from build123d import *

# Parameters (mm, degrees)
ESQUISSE1_W             = 51.5
ESQUISSE1_H             = 36.5
BOSS_EXTRU_1_DEPTH      = 5
ESQUISSE2_R             = 1.5
ENL_V_MAT_EXTRU_1_DEPTH = 5
ESQUISSE3_W             = 51.5
ESQUISSE3_H             = 2
BOSS_EXTRU_3_DEPTH      = 34.5
ESQUISSE5_R             = 1.5
ESQUISSE5_R_2           = 11
ENL_V_MAT_EXTRU_3_DEPTH = 34.5


with BuildPart() as part:
    # Esquisse1 → Boss.-Extru.1 (new body)
    with BuildSketch(Plane.XY):
        with Locations((11.117800259, -7.384341637)):
            Rectangle(ESQUISSE1_W, ESQUISSE1_H)
    extrude(amount=BOSS_EXTRU_1_DEPTH)

    # Esquisse2 → Enlèv. mat.-Extru.1 (cut)
    with BuildSketch(Plane.XY.offset(5)):
        with Locations((-10.382199741, 4.615658363)):
            Circle(ESQUISSE2_R)
        with Locations((-10.382199741, -21.384341637)):
            Circle(ESQUISSE2_R)
        with Locations((32.617800259, -21.384341637)):
            Circle(ESQUISSE2_R)
        with Locations((32.617800259, 4.615658363)):
            Circle(ESQUISSE2_R)
    extrude(amount=-ENL_V_MAT_EXTRU_1_DEPTH, mode=Mode.SUBTRACT)

    # Esquisse3 → Boss.-Extru.3 (add)
    with BuildSketch(Plane.XY.offset(5)):
        with Locations((11.117800259, 9.865658363)):
            Rectangle(ESQUISSE3_W, ESQUISSE3_H)
    extrude(amount=BOSS_EXTRU_3_DEPTH)

    # Esquisse5 → Enlèv. mat.-Extru.3 (cut)
    with BuildSketch(Plane.XZ.offset(-8.865658363)):
        with Locations((-1.882199741, 35.25)):
            Circle(ESQUISSE5_R)
        with Locations((24.117800259, 35.25)):
            Circle(ESQUISSE5_R)
        with Locations((-1.882199741, 9.25)):
            Circle(ESQUISSE5_R)
        with Locations((24.117800259, 9.25)):
            Circle(ESQUISSE5_R)
        with Locations((11.117800259, 22.25)):
            Circle(ESQUISSE5_R_2)
    extrude(amount=-ENL_V_MAT_EXTRU_3_DEPTH, mode=Mode.SUBTRACT)


solid = part.part
Model file for the job. Use its own axes, mm. A direction names the side the tool comes from. Give positions to 0.01 mm unless a question says otherwise; leave off trailing zeros. Loops run counter-clockwise (first coordinate to the right, second up) from the corner with the lowest first, then second, coordinate; pieces in that order, holes last. Notation, with made-up numbers: (4.25, 67) - (14.25, 67) arc R23 cw to (14.25, 102) - close; hole circle Ø3 at (5, 62.5). An arc over 180 degrees is marked (long way). Use one line per item in the form item = value.
(1) Pull direction X, two halves, no side cores. Call faces 3 (the face through (31.12, -21.32, 2.54)), 4 (the face through (-3.073, 9.852, 8.337)), 5 (the face through (11, -8, 5)), 6 (the face through (36.868, -5, 4)): pulls with the +X half, pulls with the -X half, needs draft (parallel to the pull), parting line crosses it, or undercut.
Determined:
face_3 = undercut
face_4 = undercut
face_5 = needs draft
face_6 = pulls with the +X half
(2) Drill centre lines: L1, parallel to X at y = 4.5, z = 4; L2, parallel to X at y = 4, z = 2; L3, parallel to Z at x = 24, y = -23. Where is each one in solid material? Low to high.
Determined:
L1 = -14.63 to -11.88, -8.89 to 31.12, 34.11 to 36.87
L2 = -14.63 to -11.75, -9.01 to 31.25, 33.99 to 36.87
L3 = 0 to 5
(3) 3-axis set-ups, long thin cutter, end or side, ignore diameter. For faces 1 (the face through (11, 10.866, 11)), 2 (the face through (-1, 8.866, 22)): which of +Z, -Z, +X, -X, +Y, -Y reach the whole face in a straight line?
Determined:
face_1 = +Z, -Z, +X, -X, +Y
face_2 = +Z, +X, -X, -Y
(4) Drop flat-ended pins along their axis: P1, Ø17, axis at x = 22, z = 14, coming from the -Y side; P2, Ø1.8, axis at x = 32.62, y = -21.38, coming from the +Z side; P3, Ø1.5, axis at x = -2, y = -10.5, coming from the +Z side. Give the stop position or say it passes through.
Determined:
P1 = 8.87
P2 = through
P3 = 5
(5) Cut at A-A (z = 22.25). Give the cut face in (x, y).
Determined:
outline = (-14.63, 8.87) - (0.12, 8.87) - (0.12, 10.87) - (-14.63, 10.87) - close; (22.12, 8.87) - (36.87, 8.87) - (36.87, 10.87) - (22.12, 10.87) - close
(6) Cut at C-C (x = 13). Give the cut face in (y, z), then the cut area to 3 significant figures.
Determined:
outline = (-25.63, 0) - (10.87, 0) - (10.87, 11.41) - (8.87, 11.41) - (8.87, 5) - (-25.63, 5) - close; (8.87, 33.09) - (10.87, 33.09) - (10.87, 39.5) - (8.87, 39.5) - close
area = 208 mm^2
(7) Cut at B-B (y = 4). Give the cut face in (x, z).
Determined:
outline = (-14.63, 0) - (-11.75, 0) - (-11.75, 5) - (-14.63, 5) - close; (-9.01, 0) - (31.25, 0) - (31.25, 5) - (-9.01, 5) - close; (33.99, 0) - (36.87, 0) - (36.87, 5) - (33.99, 5) - close
(8) Cut at D-D (z = 35.25). Give the cut face in (x, y).
Determined:
outline = (-14.63, 8.87) - (-3.38, 8.87) - (-3.38, 10.87) - (-14.63, 10.87) - close; (-0.38, 8.87) - (22.62, 8.87) - (22.62, 10.87) - (-0.38, 10.87) - close; (25.62, 8.87) - (36.87, 8.87) - (36.87, 10.87) - (25.62, 10.87) - close
